Could you check a few things on this model? Use its own coordinates, in mm. Face numbers are marked on the shaded views. A direction names the side the tool comes from. Coordinates: 2 decimals unless noted, no trailing zeros. Write each loop counter-clockwise with the first axis right and the second up, starting at its lowest first coordinate (ties: lowest second). Pieces come first, ordered by that corner, then holes.
```python
from build123d import *
from build123d.topology import SkipClean

# Parameters (mm, degrees)
EXTRUDE_1_DEPTH          = 2
CUT_EXTRUDE_3_DEPTH      = 26.250159217995726
CUT_EXTRUDE_3_DEPTH_BACK = 26.250159217995726
SKETCH_1_3_R             = 2
SKETCH_1_3_R_2           = 1.9999999999999996
FILLET_1_R               = 3
EXTRUDE_START            = -1
EXTRUDE_2_DEPTH          = 1
SKETCH_2_R               = 1.9999999999999996
EXTRUDE_3_DEPTH          = 6
SKETCH_2_3_R             = 1.7999999999999992
EXTRUDE_4_DEPTH          = 4
EXTRUDE_START_2          = -10
SKETCH_2_4_R             = 1.7999999999999992
EXTRUDE_5_DEPTH          = 4


with BuildPart() as part:
    # 草图1 → 凸台-拉伸1 (new body)
    with BuildSketch(Plane(origin=(0, 0, 0), x_dir=(0, 0, -1), z_dir=(1, 0, 0))):
        with BuildLine():
            Line((1.4791639160924377, 3.172077254628277), (-1.4791639160924381, -3.172077254628276))
            Line((-1.4791639160924381, -3.172077254628276), (3.1918530496674338, -3.172077254628276))
            ThreePointArc((3.1918530496673796, -3.172077254628116), (4.160128527071201, -1.7156137788699422), (4.5, -1.1e-15))
            ThreePointArc((4.5, 0), (4.384156275694355, 1.0144820108261179), (4.042589444315643, 1.9767322997077126))
            Line((4.042589444315688, 1.9767322997077619), (1.4791639160924377, 3.172077254628277))
        make_face()
        with BuildLine():
            Line((1.0842616121308644, -4.367422209548816), (-1.4791639160924381, -3.172077254628276))
            Line((-1.4791639160924381, -3.172077254628276), (-1.479163916092438, -4.249949894919907))
            ThreePointArc((-1.4791639160925047, -4.249949894919926), (-0.20600216890754225, -4.495282316652135), (1.0842616121308772, -4.367422209548712))
        make_face()
        with BuildLine():
            Line((3.1918530496674338, -3.172077254628276), (-1.4791639160924381, -3.172077254628276))
            Line((-1.4791639160924381, -3.172077254628276), (1.0842616121308644, -4.367422209548816))
            ThreePointArc((1.0842616121308772, -4.367422209548712), (2.220022869369828, -3.914268572731687), (3.1918530496673796, -3.172077254628116))
        make_face()
        with BuildLine():
            Line((-1.479163916092438, -4.249949894919907), (-1.4791639160924381, -3.172077254628276))
            Line((-1.4791639160924381, -3.172077254628276), (1.4791639160924377, 3.172077254628277))
            Line((1.4791639160924377, 3.172077254628277), (4.042589444315688, 1.9767322997077619))
            ThreePointArc((4.042589444315643, 1.9767322997077126), (-3.3668502191083185, 2.9856857842194757), (-1.4791639160925047, -4.249949894919926))
        make_face()
        with BuildLine():
            ThreePointArc((4.5, -1.1e-15), (4.160128527071201, -1.7156137788699422), (3.1918530496673796, -3.172077254628116))
            Line((3.1918530496674338, -3.172077254628276), (4.520836083907562, -3.172077254628276))
            Line((4.520836083907562, -3.172077254628276), (4.520836083907562, -5.969923203558247))
            Line((4.520836083907563, -5.969923203558248), (10.360395406591675, -8.692954435976247))
            ThreePointArc((10.360395406591717, -8.69295443597619), (9.969385657403148, -4.6488008791476965), (13.318723238776467, -2.3487999267197663))
            Line((13.318723238776487, -2.348799926719662), (4.042589444315688, 1.9767322997077619))
            ThreePointArc((4.042589444315643, 1.9767322997077126), (4.384156275694355, 1.0144820108261179), (4.5, 0))
        make_face()
        with BuildLine():
            Line((4.520836083907562, -3.172077254628276), (3.1918530496674338, -3.172077254628276))
            ThreePointArc((3.1918530496673796, -3.172077254628116), (2.220022869369828, -3.914268572731687), (1.0842616121308772, -4.367422209548712))
            Line((1.0842616121308644, -4.367422209548816), (4.520836083907563, -5.969923203558248))
            Line((4.520836083907562, -5.969923203558247), (4.520836083907562, -3.172077254628276))
        make_face()
        with BuildLine():
            ThreePointArc((1.0842616121308772, -4.367422209548712), (-0.20600216890754225, -4.495282316652135), (-1.4791639160925047, -4.249949894919926))
            Line((-1.479163916092438, -4.249949894919907), (-1.4791639160924364, -18))
            Line((-1.4791639160924364, -18), (4.520836083907564, -18.000000000000004))
            Line((4.520836083907564, -18.000000000000004), (4.520836083907562, -5.969923203558247))
            Line((4.520836083907563, -5.969923203558248), (1.0842616121308644, -4.367422209548816))
        make_face()
        with BuildLine():
            ThreePointArc((17.59461680554977, -6.3392739261104545), (16.323758221169964, -3.4149300452464746), (13.318723238776467, -2.3487999267197663))
            Line((13.318723238776487, -2.348799926719663), (15.073780721642205, -3.1671966714821758))
            Line((15.073780721642205, -3.167196671482176), (12.115452889457329, -9.51135118073873))
            Line((12.115452889457327, -9.51135118073873), (10.360395406591675, -8.692954435976247))
            ThreePointArc((10.360395406591717, -8.69295443597619), (14.832177794787833, -10.143014558424401), (17.59461680554977, -6.339273926110455))
        make_face()
        with BuildLine():
            Line((15.073780721642205, -3.1671966714821758), (13.318723238776487, -2.348799926719663))
            ThreePointArc((13.318723238776467, -2.3487999267197663), (9.969385657403148, -4.6488008791476965), (10.360395406591717, -8.69295443597619))
            Line((10.360395406591675, -8.692954435976247), (12.115452889457327, -9.51135118073873))
            Line((12.115452889457329, -9.51135118073873), (15.073780721642205, -3.167196671482176))
        make_face()
    extrude(amount=EXTRUDE_1_DEPTH)

    # 草图1<3> → 切除-拉伸3 (cut, two sides: drawn at the far end of the back side and taken through both)
    with BuildSketch(Plane(origin=(0, 0, 0), x_dir=(0, 0, -1), z_dir=(1, 0, 0)).offset(-CUT_EXTRUDE_3_DEPTH_BACK)):
        Circle(SKETCH_1_3_R)
        with Locations((13.594616805549768, -6.3392739261104545)):
            Circle(SKETCH_1_3_R_2)
    extrude(amount=CUT_EXTRUDE_3_DEPTH + CUT_EXTRUDE_3_DEPTH_BACK, mode=Mode.SUBTRACT)

    # 圆角1
    fillet_1_edges = [part.edges().sort_by_distance(p)[0] for p in [
        (1, -2.3487999267197144, -13.318723238776478),
        (1, 1.9767322997077375, -4.0425894443156665),
        (1, -8.692954435976219, -10.360395406591696),
        (1, -5.969923203558247, -4.520836083907563),
        (1, -4.249949894919917, 1.4791639160924714),
    ]]
    fillet(fillet_1_edges, radius=FILLET_1_R)

    # 草图1<4> → 凸台-拉伸2 (add)
    with SkipClean():  # the faces are left unmerged after this step: merging them gives an invalid solid
        with BuildSketch(Plane(origin=(0, 0, 0), x_dir=(0, 0, -1), z_dir=(1, 0, 0)).offset(EXTRUDE_START)):
            with BuildLine():
                ThreePointArc((17.59461680554977, -6.3392739261104545), (16.323758221169964, -3.4149300452464746), (13.318723238776467, -2.3487999267197663))
                Line((13.318723238776487, -2.348799926719663), (15.073780721642205, -3.1671966714821758))
                Line((15.073780721642205, -3.167196671482176), (14.43985332903116, -4.526658352037151))
                ThreePointArc((14.439853329031175, -4.526658352037159), (15.28139969717554, -5.264674709416811), (15.594616805549768, -6.3392739261104545))
                ThreePointArc((15.594616805549768, -6.339273926110455), (14.66921602224341, -8.02605681773623), (12.749380282068358, -8.15188950018375))
                Line((12.749380282068373, -8.151889500183756), (12.115452889457329, -9.51135118073873))
                Line((12.115452889457327, -9.51135118073873), (10.360395406591675, -8.692954435976247))
                ThreePointArc((10.360395406591717, -8.69295443597619), (14.832177794787833, -10.143014558424401), (17.59461680554977, -6.339273926110455))
            make_face()
            with BuildLine():
                Line((15.073780721642205, -3.1671966714821758), (13.318723238776487, -2.348799926719663))
                ThreePointArc((13.318723238776467, -2.3487999267197663), (9.969385657403148, -4.6488008791476965), (10.360395406591717, -8.69295443597619))
                Line((10.360395406591675, -8.692954435976247), (12.115452889457327, -9.51135118073873))
                Line((12.115452889457329, -9.51135118073873), (12.749380282068373, -8.151889500183756))
                ThreePointArc((12.749380282068358, -8.15188950018375), (11.782001231476473, -5.494037402629046), (14.439853329031175, -4.526658352037159))
                Line((14.43985332903116, -4.526658352037151), (15.073780721642205, -3.167196671482176))
            make_face()
        extrude(amount=EXTRUDE_2_DEPTH)

    # 镜向1: part across plane


with BuildPart() as part_1:
    with SkipClean():  # the faces are left unmerged after this step: merging them gives an invalid solid
        add(part.part)
        add(part.part.mirror(Plane.ZY.offset(1)))

    # 草图2 → 凸台-拉伸3 (add)
    with BuildSketch(Plane(origin=(2, 0, 0), x_dir=(0, 0, -1), z_dir=(1, 0, 0))):
        with Locations((13.594616805549768, -6.3392739261104545)):
            Circle(SKETCH_2_R)
    extrude(amount=-EXTRUDE_3_DEPTH)

    # 草图2<3> → 凸台-拉伸4 (add)
    with BuildSketch(Plane(origin=(2, 0, 0), x_dir=(0, 0, -1), z_dir=(1, 0, 0))):
        with Locations((13.594616805549768, -6.3392739261104545)):
            Circle(SKETCH_2_3_R)
    extrude(amount=EXTRUDE_4_DEPTH)

    # 草图2<4> → 凸台-拉伸5 (add)
    with BuildSketch(Plane(origin=(2, 0, 0), x_dir=(0, 0, -1), z_dir=(1, 0, 0)).offset(EXTRUDE_START_2)):
        with Locations((13.594616805549768, -6.3392739261104545)):
            Circle(SKETCH_2_4_R)
    extrude(amount=EXTRUDE_5_DEPTH)


solid = part_1.part
```
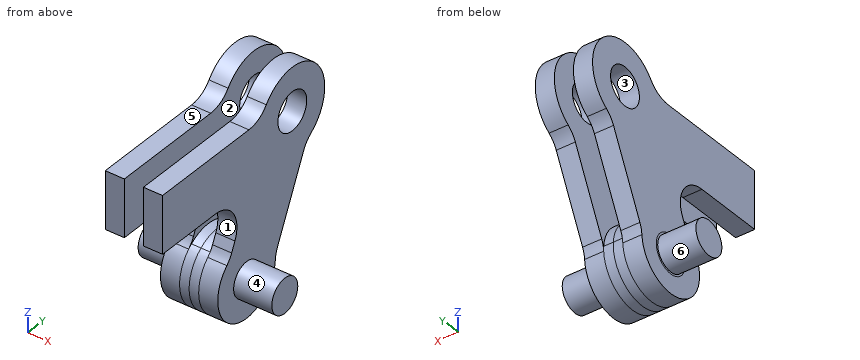
1. Please list where these lines run through material, in increasing order: line 1 along X through (y, z) = (-1, -6); line 2 along Y through (x, z) = (-3.1, 0); line 3 along Z through (x, y) = (-2.5, -0.75).
Verdict:
line 1: x = -4 to -2, 0 to 2
line 2: y = -18 to -2, 2 to 4.5
line 3: z = -9.89 to -1.85, 1.85 to 4.44
2. On a 3-axis mill with a long thin cutter (end or side, diameter ignored), from which of +Z, -Z, +X, -X, +Y, -Y can I reach the whole of each face in a straight line? I mean the marked faces 4, 5 and 6. Say none if no direction works.
Verdict:
face 4: +X
face 5: +Z, +X, -X, -Y
face 6: -X
3. I want a section at B-B on z = 0. Please give me the cut outline in (x, y), plus the area to 3 significant figures.
Verdict:
outline: (-4, -18) - (-2, -18) - (-2, -2) - (-4, -2) - close; (-4, 2) - (-2, 2) - (-2, 4.5) - (-4, 4.5) - close; (0, -18) - (2, -18) - (2, -2) - (0, -2) - close; (0, 2) - (2, 2) - (2, 4.5) - (0, 4.5) - close
area: 74.0 mm2
4. I want a section at D-D on y = 0. Please give me the cut outline in (x, z).
Verdict:
outline: (-4, -8.28) - (-2, -8.28) - (-2, -2) - (-4, -2) - close; (-4, 2) - (-2, 2) - (-2, 4.5) - (-4, 4.5) - close; (0, -8.28) - (2, -8.28) - (2, -2) - (0, -2) - close; (0, 2) - (2, 2) - (2, 4.5) - (0, 4.5) - close
5. I want a section at C-C on x = 1.25. Please give me the cut outline in (y, z), plus the area to 3 significant figures.
Verdict:
outline: (-18, -4.52) - (-10.68, -4.52) arc R3 cw to (-7.96, -8.79) - (-8.41, -9.76) arc R3 cw to (-9.08, -10.68) arc R4 ccw (long way) to (-2.35, -13.82) arc R3 cw to (-2.07, -12.72) - (1.59, -4.87) arc R3 cw to (2.59, -3.68) arc R4.5 ccw (long way) to (-3.61, 2.69) arc R3 cw to (-6.02, 1.48) - (-18, 1.48) - close; hole circle Ø4 at (0, 0)
area: 239 mm2
6. If we mould it in two halves opening along Y, with no side actions, what happens to the marked faces 1, 2 and 3? For each: pulls with the +Y half, pulls with the -Y half, needs draft (parallel to the pull), parting line crosses it, or undercut.
Verdict:
face 1: pulls with the -Y half
face 2: needs draft
face 3: undercut
7. For pin 1 (4 mm diameter, centred on x = 1.5, z = -6.5, fed in from +Y); pin 2 (2.5 mm diameter, centred on y = 0, z = 0, fed in from -X); pin 3 (2 mm diameter, centred on x = -2.5, y = -15.5, fed in from -Z); pin 4 (8 mm diameter, centred on x = 1, z = -12, fed in from -Y), each with a flat end and sliding along its axis, tell me the tip position at first contact or that it passes through.
Verdict:
pin 1: stops at y = 1.8
pin 2: passes through
pin 3: stops at z = -4.52
pin 4: stops at y = -10.34
8. I want a section at A-A on y = -16. Please give me the cut outline in (x, z), plus the area to 3 significant figures.
Verdict:
outline: (-4, -4.52) - (-2, -4.52) - (-2, 1.48) - (-4, 1.48) - close; (0, -4.52) - (2, -4.52) - (2, 1.48) - (0, 1.48) - close
area: 24.0 mm2
